Verification items for the finished model (mm, model axes). A direction names the side the tool comes from. Give positions to 0.01 mm unless a question says otherwise; leave off trailing zeros. Write each loop counter-clockwise with the first axis right and the second up, starting at its lowest first coordinate (ties: lowest second). Pieces come first, ordered by that corner, then holes. Notation, with made-up numbers: (4.25, 21) -> (13.25, 21) arc R20 ccw to (13.25, 60) -> close; hole circle Ø7 at (87.25, 86). An arc over 180 degrees is marked (long way). Answer as CSV lines item,"result".
```python
from build123d import *

# Parameters (mm, degrees)
CROQUIS1_R              = 11.05
SALIENTE_EXTRUIR2_DEPTH = 6
CROQUIS3_R              = 9.7
CORTAR_EXTRUIR2_DEPTH   = 6
CROQUIS7_R              = 2.94693617
CROQUIS7_R_2            = 2.946936168
CORTAR_EXTRUIR3_DEPTH   = 10.56
CROQUIS8_W              = 2.7
CROQUIS8_H              = 1.7
REDONDEO1_R             = 0.5
CROQUIS9_W              = 1.8
CROQUIS9_H              = 5.1
CORTAR_EXTRUIR7_START   = -0.4
CROQUIS14_R             = 6.45
CROQUIS14_R_2           = 6.3
CORTAR_EXTRUIR7_DEPTH   = 0.4
CORTAR_EXTRUIR8_DEPTH   = 0.7


with BuildPart() as part:
    # Croquis1 → Saliente-Extruir2 (new body)
    with BuildSketch(Plane(origin=(0, 0, 0), x_dir=(1, 0, 0), z_dir=(0, 1, 0))):
        with Locations(Location((0, 0, 0), (0, 0, 270))):
            Circle(CROQUIS1_R)
    extrude(amount=SALIENTE_EXTRUIR2_DEPTH)

    # Croquis3 → Cortar-Extruir2 (cut)
    with BuildSketch(Plane(origin=(0, 6, 0), x_dir=(1, 0, 0), z_dir=(0, 1, 0))):
        with Locations(Location((0, 0, 0), (0, 0, 270))):
            Circle(CROQUIS3_R)
    extrude(amount=-CORTAR_EXTRUIR2_DEPTH, mode=Mode.SUBTRACT)

    # Croquis4 → Revolución1 (revolve)
    with BuildSketch(Plane.XY, mode=Mode.PRIVATE) as revoluci_n1_sk:
        with BuildLine():
            Line((6.05, 9.65), (6.05, 11))
            ThreePointArc((6.05, 11), (9.585533906, 9.535533906), (11.05, 6))
            Line((11.05, 6), (9.7, 6))
            ThreePointArc((9.7, 6), (8.630939751, 8.580939751), (6.05, 9.65))
        make_face()
    revolve(revoluci_n1_sk.sketch.rotate(Axis((0, 0, 0), (0, 1, 0)), 90), axis=Axis((0, 0, 0), (0, 1, 0)))

    # Croquis7 → Cortar-Extruir3 (cut)
    with BuildSketch(Plane.XZ):
        with Locations((0, 13.34693617)):
            Circle(CROQUIS7_R)
        with Locations((-9.437709072, 9.437709072)):
            Circle(CROQUIS7_R_2)
        with Locations((9.437709074, 9.437709074)):
            Circle(CROQUIS7_R)
        with Locations((13.34693617, 0)):
            Circle(CROQUIS7_R)
        with Locations((9.437709074, -9.437709074)):
            Circle(CROQUIS7_R)
        with Locations((0, -13.34693617)):
            Circle(CROQUIS7_R)
        with Locations((-9.437709074, -9.437709074)):
            Circle(CROQUIS7_R)
        with Locations((-13.34693617, 0)):
            Circle(CROQUIS7_R)
    extrude(amount=-CORTAR_EXTRUIR3_DEPTH, mode=Mode.SUBTRACT)

    # Croquis8 → Revolución2 (revolve)
    with BuildSketch(Plane.XY, mode=Mode.PRIVATE) as revoluci_n2_sk:
        with Locations((-6, 11.665880959)):
            Rectangle(CROQUIS8_W, CROQUIS8_H)
    revolve(revoluci_n2_sk.sketch.rotate(Axis((0, 0, 0), (0, 1, 0)), 270), axis=Axis((0, 0, 0), (0, 1, 0)))

    # Redondeo1
    redondeo1_edges = [part.edges().sort_by_distance(p)[0] for p in [
        (0, 12.515880959, 7.35),
    ]]
    fillet(redondeo1_edges, radius=REDONDEO1_R)

    # Croquis9 → Revolución3 (revolve)
    with BuildSketch(Plane.XY, mode=Mode.PRIVATE) as revoluci_n3_sk:
        with Locations((-5.55, 15.065880959)):
            Rectangle(CROQUIS9_W, CROQUIS9_H)
    revolve(revoluci_n3_sk.sketch.rotate(Axis((0, 0, 0), (0, 1, 0)), 270), axis=Axis((0, 0, 0), (0, 1, 0)))

    # Croquis14 → Cortar-Extruir7 (cut)
    with BuildSketch(Plane(origin=(0, 17.615880959, 0), x_dir=(1, 0, 0), z_dir=(0, 1, 0)).offset(CORTAR_EXTRUIR7_START)):
        with Locations(Location((0, 0, 0), (0, 0, 90))):
            Circle(CROQUIS14_R)
        with Locations(Location((0, 0, 0), (0, 0, 270))):
            Circle(CROQUIS14_R_2, mode=Mode.SUBTRACT)
    extrude(amount=CORTAR_EXTRUIR7_DEPTH, mode=Mode.SUBTRACT)

    # Croquis10 → Cortar-Extruir8 (cut)
    with BuildSketch(Plane(origin=(0, 17.615880959, 0), x_dir=(1, 0, 0), z_dir=(0, 1, 0))):
        with BuildLine():
            Line((-6.45, -0.5), (-5.22613624, -0.5))
            ThreePointArc((-5.22613624, -0.5), (0, -5.25), (5.22613624, -0.5))
            Line((5.22613624, -0.5), (6.45, -0.5))
            Line((6.45, -0.5), (6.45, 0.5))
            Line((6.45, 0.5), (5.22613624, 0.5))
            ThreePointArc((5.22613624, 0.5), (0, 5.25), (-5.22613624, 0.5))
            Line((-5.22613624, 0.5), (-6.45, 0.5))
            Line((-6.45, 0.5), (-6.45, -0.5))
        make_face()
    extrude(amount=-CORTAR_EXTRUIR8_DEPTH, mode=Mode.SUBTRACT)


solid = part.part
```
1) Scan lines: line 1 along X through (y, z) = (13, 0); line 2 along X through (y, z) = (2, 0); line 3 along Y through (x, z) = (-4.75, -3.5). Record each from-to range of solid material in increasing order.
Reported:
line 1,"-6.45 to -4.65, 4.65 to 6.45"
line 2,"-10.4 to -9.7, 9.7 to 10.4"
line 3,"10.82 to 17.62"
2) Depth check by flat-ended pin: pin 1 (5 mm diameter, centred on y = 6, z = -1.5, fed in from -X); pin 2 (8 mm diameter, centred on x = -3, y = 11.5, fed in from +Z); pin 3 (1.5 mm diameter, centred on y = 10.5, z = -3.5, fed in from +X); pin 4 (2 mm diameter, centred on y = 6, z = -7, fed in from +X). Enter the tip coordinate at first touch or a pass-through.
Reported:
pin 1,"x = -10.92"
pin 2,"z = 10.61"
pin 3,"x = 8.72"
pin 4,"x = 9.28"
3) Tool access check on faces 4 (the flat face through (4.5, 10.816, -1.8)), 5 (the cylindrical face through (-10.4, 4.2, 0)), 6 (the flat face through (10, 0, -1)), 7 (the cylindrical face through (0.1, 17.4, -6.3)), 8 (the cylindrical face through (7.175, 11.43, 1.593)). Record the directions out of +Z, -Z, +X, -X, +Y, -Y that give a thin tool (end or side, any length) a straight path to the whole face; none if there is none.
Reported:
face 4,"-Y"
face 5,"-X, +Y, -Y"
face 6,"+Z, -Z, +X, -X, -Y"
face 7,"-Z, +Y"
face 8,"+Y"
4) Section check B-B (z = 0). Record the boundary of the cut face in (x, y), and give its area (3 significant figures).
Reported:
outline,"(-10.4, 0) -> (-9.7, 0) -> (-9.7, 6) arc R3.65 cw to (-6.05, 9.65) -> (-6.05, 10.82) -> (-4.65, 10.82) -> (-4.65, 16.92) -> (-6.45, 16.92) -> (-6.45, 12.52) -> (-6.85, 12.52) arc R0.5 ccw to (-7.35, 12.02) -> (-7.35, 10.83) arc R5 ccw to (-10.4, 8.47) -> close; (4.65, 10.82) -> (6.05, 10.82) -> (6.05, 9.65) arc R3.65 cw to (9.7, 6) -> (9.7, 0) -> (10.4, 0) -> (10.4, 8.47) arc R5 ccw to (7.35, 10.83) -> (7.35, 12.02) arc R0.5 ccw to (6.85, 12.52) -> (6.45, 12.52) -> (6.45, 16.92) -> (4.65, 16.92) -> close"
area,"49.2 mm²"
5) Draft check along X on faces 1 (the cylindrical face through (-0.1, 17.4, 6.3)), 2 (the cylindrical face through (-7.34, 4.18, -7.37)), 3 (the cylindrical face through (-1.82, 10.24, -5.77)). Enter one of: +X half, -X half, draft (parallel to the pull), parting line (faces both ways), or undercut.
Reported:
face 1,"parting line"
face 2,"-X half"
face 3,"undercut"
6) Section check C-C (y = 2.5). Record the boundary of the cut face in (x, z) (3 decimals).
Reported:
outline,"(-10.922, -1.675) arc R11.05 ccw to (-8.908, -6.539) arc R2.947 cw to (-6.539, -8.908) arc R11.05 ccw to (-1.675, -10.922) arc R2.947 cw to (1.675, -10.922) arc R11.05 ccw to (6.539, -8.908) arc R2.947 cw to (8.908, -6.539) arc R11.05 ccw to (10.922, -1.675) arc R2.947 cw to (10.922, 1.675) arc R11.05 ccw to (8.908, 6.539) arc R2.947 cw to (6.539, 8.908) arc R11.05 ccw to (1.675, 10.922) arc R2.947 cw to (-1.675, 10.922) arc R11.05 ccw to (-6.539, 8.908) arc R2.947 cw to (-8.908, 6.539) arc R11.05 ccw to (-10.922, 1.675) arc R2.947 cw to start; hole circle Ø19.4 at (0, 0)"
7) Section check D-D (y = 11.5). Record the boundary of the cut face in (x, z), and give its area (3 significant figures).
Reported:
outline,"circle Ø14.7 at (0, 0); hole circle Ø9.3 at (0, 0)"
area,"102 mm²"
